Verification items for the finished model (mm, model axes). Face numbers are marked on the shaded views. A direction names the side the tool comes from. Give positions to 0.01 mm unless a question says otherwise; leave off trailing zeros. Loops run counter-clockwise (first coordinate to the right, second up) from the corner with the lowest first, then second, coordinate; pieces in that order, holes last. Notation, with made-up numbers: M 27,19 L 53,19 A21 cw 53,51 Z; hole C 49.5,-2.5 d6. An arc over 180 degrees is marked long. Use CSV: the item, a comma, the result in double quotes.
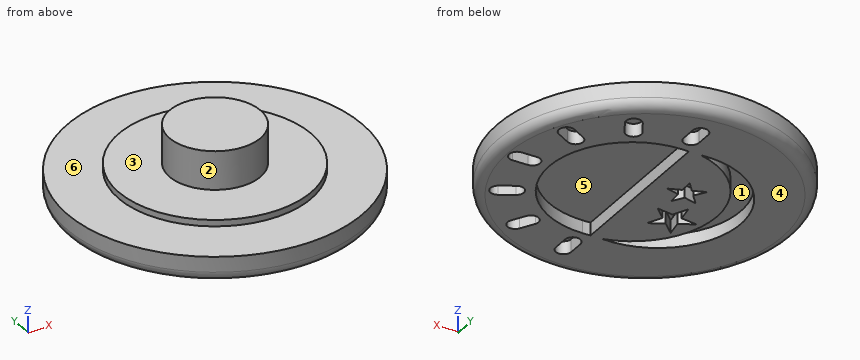
from build123d import *

# Parameters (mm, degrees)
F0_R     = 11.5
F1_DEPTH = 2
F2_R     = 7.5
F3_DEPTH = 0.5
F4_R     = 3.55
F5_DEPTH = 3
F7_DEPTH = 1
F8_R     = 0.8


with BuildPart() as f1:
    # F0 (on Top) → F1 (new body)
    with BuildSketch(Plane.XY):
        Circle(F0_R)
    extrude(amount=F1_DEPTH)

    # F2 (on face) → F3 (join)
    with BuildSketch(Plane.XY.offset(2)):
        Circle(F2_R)
    extrude(amount=F3_DEPTH)

    # F4 (on face) → F5 (join)
    with BuildSketch(Plane.XY.offset(2.5)):
        Circle(F4_R)
    extrude(amount=F5_DEPTH)

    # F6 (on face) → F7 (cut)
    with BuildSketch(Plane(origin=(0, 0, 0), x_dir=(1, 0, 0), z_dir=(0, 0, -1))):
        with BuildLine():
            ThreePointArc((-0.4961662294, -6.4166546046), (-5.5796541594, 0), (-0.4961662294, 6.4166546046))
            ThreePointArc((-0.4961662294, 6.4166546046), (-7.4491550771, 0), (-0.4961662294, -6.4166546046))
        make_face()
        with BuildLine():
            Line((1.6118148057, 7.7430446076), (1.6118148057, 8.9430446076))
            ThreePointArc((1.6118148057, 8.9430446076), (1.0118148057, 9.5430446076), (0.4118148057, 8.9430446076))
            Line((0.4118148057, 8.9430446076), (0.4118148057, 7.7430446076))
            ThreePointArc((0.4118148057, 7.7430446076), (1.0118148057, 7.1430446076), (1.6118148057, 7.7430446076))
        make_face()
        with BuildLine():
            ThreePointArc((1.6118148057, -7.7430446076), (1.0118148057, -7.1430446076), (0.4118148057, -7.7430446076))
            Line((0.4118148057, -7.7430446076), (0.4118148057, -8.9430446076))
            ThreePointArc((0.4118148057, -8.9430446076), (1.0118148057, -9.5430446076), (1.6118148057, -8.9430446076))
            Line((1.6118148057, -8.9430446076), (1.6118148057, -7.7430446076))
        make_face()
        with BuildLine():
            ThreePointArc((1.0118148057, 6.4373402714), (0.7114877838, 6.4303307418), (0.4118148057, 6.4093174184))
            Line((0.4118148057, 6.4093174184), (0.4118148057, -6.4093174184))
            ThreePointArc((0.4118148057, -6.4093174184), (0.7114877838, -6.4303307418), (1.0118148057, -6.4373402714))
            Line((1.0118148057, -6.4373402714), (1.0118148057, 6.4373402714))
        make_face()
        with BuildLine():
            ThreePointArc((1.0118148057, -6.4373402714), (7.4491550771, 0), (1.0118148057, 6.4373402714))
            Line((1.0118148057, 6.4373402714), (1.0118148057, -6.4373402714))
        make_face()
        with BuildLine():
            Line((4.9637218672, 8.0449038174), (4.3637218672, 7.0056733328))
            ThreePointArc((4.3637218672, 7.0056733328), (4.5833371095, 6.1860580905), (5.4029523517, 6.4056733328))
            Line((5.4029523517, 6.4056733328), (6.0029523517, 7.4449038174))
            ThreePointArc((6.0029523517, 7.4449038174), (5.7833371095, 8.2645190596), (4.9637218672, 8.0449038174))
        make_face()
        with BuildLine():
            Line((8.456718623, 4.9911375461), (7.4174881385, 4.3911375461))
            ThreePointArc((7.4174881385, 4.3911375461), (7.1978728962, 3.5715223038), (8.0174881385, 3.3519070615))
            Line((8.0174881385, 3.3519070615), (9.056718623, 3.9519070615))
            ThreePointArc((9.056718623, 3.9519070615), (9.2763338653, 4.7715223038), (8.456718623, 4.9911375461))
        make_face()
        with BuildLine():
            Line((9.9548594133, 0.6), (8.7548594133, 0.6))
            ThreePointArc((8.7548594133, 0.6), (8.1548594133, 0), (8.7548594133, -0.6))
            Line((8.7548594133, -0.6), (9.9548594133, -0.6))
            ThreePointArc((9.9548594133, -0.6), (10.5548594133, 0), (9.9548594133, 0.6))
        make_face()
        with BuildLine():
            Line((9.056718623, -3.9519070615), (8.0174881385, -3.3519070615))
            ThreePointArc((8.0174881385, -3.3519070615), (7.1978728962, -3.5715223038), (7.4174881385, -4.3911375461))
            Line((7.4174881385, -4.3911375461), (8.456718623, -4.9911375461))
            ThreePointArc((8.456718623, -4.9911375461), (9.2763338653, -4.7715223038), (9.056718623, -3.9519070615))
        make_face()
        with BuildLine():
            Line((6.0029523517, -7.4449038174), (5.4029523517, -6.4056733328))
            ThreePointArc((5.4029523517, -6.4056733328), (4.5833371095, -6.1860580905), (4.3637218672, -7.0056733328))
            Line((4.3637218672, -7.0056733328), (4.9637218672, -8.0449038174))
            ThreePointArc((4.9637218672, -8.0449038174), (5.7833371095, -8.2645190596), (6.0029523517, -7.4449038174))
        make_face()
        Polygon((-3.8030603375, 2.1452946133), (-4.9306933834, 1.548157713), (-3.6674308223, 1.368445539), align=None)
        Polygon((-4.022513503, 3.4022628198), (-3.8030603375, 2.1452946133), (-3.1061447883, 2.5143455137), align=None)
        Polygon((-3.1061447883, 2.5143455137), (-3.8030603375, 2.1452946133), (-3.6674308223, 1.368445539), (-2.8866916228, 1.2573773072), (-2.5397977764, 1.9655824393), align=None)
        Polygon((-2.8866916228, 1.2573773072), (-3.6674308223, 1.368445539), (-3.4479776567, 0.1114773325), align=None)
        Polygon((-1.9785117424, 3.1114824139), (-3.1061447883, 2.5143455137), (-2.5397977764, 1.9655824393), align=None)
        Polygon((-2.5397977764, 1.9655824393), (-2.8866916228, 1.2573773072), (-1.6234290616, 1.0776651331), align=None)
        Polygon((-2.8006232783, -1.6000521775), (-3.3599715105, -2.463868964), (-2.3997105171, -2.0938031454), align=None)
        Polygon((-3.4493137525, -0.8011463294), (-2.8006232783, -1.6000521775), (-2.4549270593, -1.0661840434), align=None)
        Polygon((-2.4549270593, -1.0661840434), (-2.8006232783, -1.6000521775), (-2.3997105171, -2.0938031454), (-1.8062365852, -1.8650898915), (-1.840362285, -1.2299863589), align=None)
        Polygon((-1.8062365852, -1.8650898915), (-2.3997105171, -2.0938031454), (-1.7510200429, -2.8927089935), align=None)
        Polygon((-1.8955788272, -0.2023672569), (-2.4549270593, -1.0661840434), (-1.840362285, -1.2299863589), align=None)
        Polygon((-1.840362285, -1.2299863589), (-1.8062365852, -1.8650898915), (-0.8459755918, -1.4950240729), align=None)
    extrude(amount=-F7_DEPTH, mode=Mode.SUBTRACT)

    # F8
    f8_edges = [f1.edges().sort_by_distance(p)[0] for p in [
        (-11.5, 0, 0),
    ]]
    fillet(f8_edges, radius=F8_R)


solid = f1.part
(1) Mould release check, pull along Y, two halves, no side actions. Record for the marked faces 1, 2 and 3: released by +Y, released by -Y, zero draft, split by the parting line, or undercut.
Calculated:
face 1,"undercut"
face 2,"split by the parting line"
face 3,"zero draft"
(2) Scan lines: L1, parallel to X at y = -7.25, z = 0.9; L2, parallel to Y at x = -4.5, z = 0.5; L3, parallel to Z at x = 1, y = 5. Record each from-to range of solid material in increasing order. Write a range as from..to.
Calculated:
L1,"x = -8.93..0.67, 1.35..4.5, 5.89..8.93"
L2,"y = -10.52..-5.41, -3.61..-1.78, -1.49..3.61, 5.41..10.52"
L3,"z = 1..2.5"
(3) Tool access check on the marked faces 4, 5 and 6. Record the directions out of +Z, -Z, +X, -X, +Y, -Y that give a thin tool (end or side, any length) a straight path to the whole face; none if there is none.
Calculated:
face 4,"-Z, +X, -X, +Y, -Y"
face 5,"-Z"
face 6,"+Z"
(4) Depth check by flat-ended pin: pin 1 Ø0.8 at (x, z) = (9.5, 0.5) entering from +Y; pin 2 Ø1.1 at (y, z) = (-3, 0.5) entering from +X; pin 3 Ø0.6 at (x, y) = (1, 8.5) entering from -Z. Enter the tip coordinate at first touch or a pass-through.
Calculated:
pin 1,"stops at y = 6.97"
pin 2,"stops at x = 11.22"
pin 3,"stops at z = 1"
(5) Section check A-A on x = 0. Record the cut outline in (y, z), plus the area to 3 significant figures.
Calculated:
outline,"M -11.5,0.8 A0.8 ccw -10.7,0 L 10.7,0 A0.8 ccw 11.5,0.8 L 11.5,2 L 7.5,2 L 7.5,2.5 L 3.55,2.5 L 3.55,5.5 L -3.55,5.5 L -3.55,2.5 L -7.5,2.5 L -7.5,2 L -11.5,2 Z"
area,"74.5 mm²"
(6) Section check B-B on z = 2.95. Record the cut outline in (x, y), plus the area to 3 significant figures.
Calculated:
outline,"C 0,0 d7.1"
area,"39.6 mm²"
